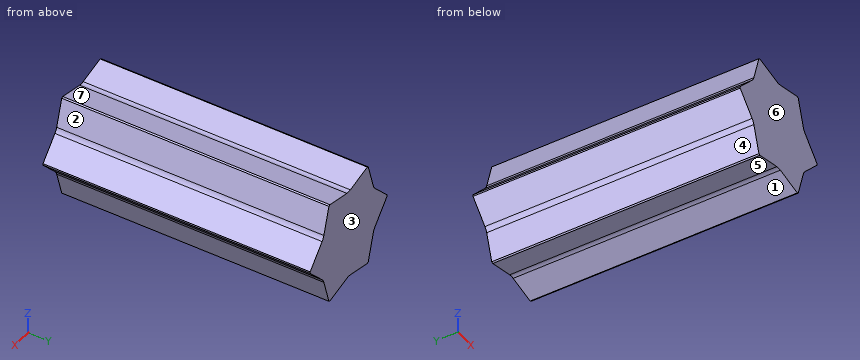
from build123d import *

# Parameters (mm, degrees)
EXTRUDE_1_DEPTH = 1480


with BuildPart() as part:
    # 草图7 → 凸台-拉伸1 (new body)
    with BuildSketch(Plane(origin=(0, 0, 0), x_dir=(1, 0, 0), z_dir=(0, 1, 0))):
        with BuildLine():
            Line((-163.425407286, 292.470977468), (-171.574592714, 287.766043068))
            Line((-171.574592714, 287.766043068), (-215.64921864, 142.144339856))
            ThreePointArc((-215.64921864, 142.144339856), (-221.758129252, 128.033988921), (-230.922998757, 115.687898132))
            Line((-230.922998757, 115.687898132), (-335, 4.7049344))
            Line((-335, 4.7049344), (-335, -4.7049344))
            Line((-335, -4.7049344), (-230.92521864, -115.68553172))
            ThreePointArc((-230.92521864, -115.68553172), (-221.75975158, -128.031178968), (-215.650158071, -142.141234176))
            Line((-215.650158071, -142.141234176), (-171.574592714, -287.766043068))
            Line((-171.574592714, -287.766043068), (-163.425407286, -292.470977468))
            Line((-163.425407286, -292.470977468), (-15.276, -257.829871576))
            ThreePointArc((-15.276, -257.829871576), (-0.001622327, -256.065167889), (15.272840686, -257.829132308))
            Line((15.272840686, -257.829132308), (163.425407286, -292.470977468))
            Line((163.425407286, -292.470977468), (171.574592714, -287.766043068))
            Line((171.574592714, -287.766043068), (215.64921864, -142.144339856))
            ThreePointArc((215.64921864, -142.144339856), (221.758129252, -128.033988921), (230.922998757, -115.687898132))
            Line((230.922998757, -115.687898132), (335, -4.7049344))
            Line((335, -4.7049344), (335, 4.7049344))
            Line((335, 4.7049344), (230.92521864, 115.68553172))
            ThreePointArc((230.92521864, 115.68553172), (221.75975158, 128.031178968), (215.650158071, 142.141234176))
            Line((215.650158071, 142.141234176), (171.574592714, 287.766043068))
            Line((171.574592714, 287.766043068), (163.425407286, 292.470977468))
            Line((163.425407286, 292.470977468), (15.276, 257.829871576))
            ThreePointArc((15.276, 257.829871576), (0.001622327, 256.065167889), (-15.272840686, 257.829132308))
            Line((-15.272840686, 257.829132308), (-163.425407286, 292.470977468))
        make_face()
    extrude(amount=EXTRUDE_1_DEPTH)


solid = part.part
Here's how the part is built. I have some questions about the finished solid (model axes, mm). Face numbers are marked on the shaded views. A direction names the side the tool comes from. Give positions to 0.01 mm unless a question says otherwise; leave off trailing zeros. Write each loop counter-clockwise with the first axis right and the second up, starting at its lowest first coordinate (ties: lowest second). Pieces come first, ordered by that corner, then holes. Notation, with made-up numbers: (-33, 46.5) -> (9, 46.5) arc R9 ccw to (9, 58.5) -> close; hole circle Ø1 at (74.25, 14). An arc over 180 degrees is marked (long way). Use one line per item in the form item = value. Start each with the question number.
1. Imagine slicing it at B-B on x = -257. List the corners of the cut face in (y, z) for me, plus the area to 3 significant figures.
2. Imagine slicing it at C-C on z = 237.5. List the corners of the cut face in (x, y) for me.
3. Thinking about a two-plate mould opening in X: for the marked faces 1, 2, 3 and 4, which applies, +X half, -X half, draft (parallel to the pull), parting line (faces both ways), or undercut?
4. On a 3-axis mill with a long thin cutter (end or side, diameter ignored), from which of +Z, -Z, +X, -X, +Y, -Y can I reach the whole of each face in a straight line? I mean the marked faces 5, 6 and 7. Say none if no direction works.
5. Imagine slicing it at A-A on y = 864. List the corners of the cut face in (x, z) for me.
6. Will these pins go through, and if not, where does the flat tip stop? pin 1 Ø5 at (y, z) = (846, 106) entering from +X; pin 2 Ø3 at (x, y) = (-232, 1296.5) entering from -Z; pin 3 Ø1 at (y, z) = (1138.5, 119) entering from +X.
7. If I drill on L1, parallel to X at y = 628.5, z = 78.5; L2, parallel to Z at x = -45, y = 397.5; L3, parallel to X at y = 1015.5, z = 165.5, over which ranges is the centre line in solid material (lowest first)?
Entries:
q1.outline = (0, -87.88) -> (1480, -87.88) -> (1480, 87.88) -> (0, 87.88) -> close
q1.area = 260,000 mm²
q2.outline = (-186.79, 0) -> (186.79, 0) -> (186.79, 1480) -> (-186.79, 1480) -> close
q3.face_1 = undercut
q3.face_2 = +X half
q3.face_3 = draft
q3.face_4 = -X half
q4.face_5 = -Z, +Y, -Y
q4.face_6 = +Z, -Z, +X, -X, -Y
q4.face_7 = +Z, +Y, -Y
q5.outline = (-335, -4.7) -> (-230.92, -115.69) arc R67 cw to (-215.65, -142.14) -> (-171.57, -287.77) -> (-163.43, -292.47) -> (-15.27, -257.83) arc R67 cw to (15.28, -257.83) -> (163.43, -292.47) -> (171.57, -287.77) -> (215.65, -142.14) arc R67 cw to (230.93, -115.69) -> (335, -4.7) -> (335, 4.7) -> (230.92, 115.69) arc R67 cw to (215.65, 142.14) -> (171.57, 287.77) -> (163.43, 292.47) -> (15.27, 257.83) arc R67 cw to (-15.28, 257.83) -> (-163.43, 292.47) -> (-171.57, 287.77) -> (-215.65, 142.14) arc R67 cw to (-230.93, 115.69) -> (-335, 4.7) -> close
q6.pin_1 = 242.35
q6.pin_2 = -116.14
q6.pin_3 = 228.43
q7.L1 = -265.8 to 265.8
q7.L2 = -264.78 to 264.78
q7.L3 = -208.58 to 208.58
